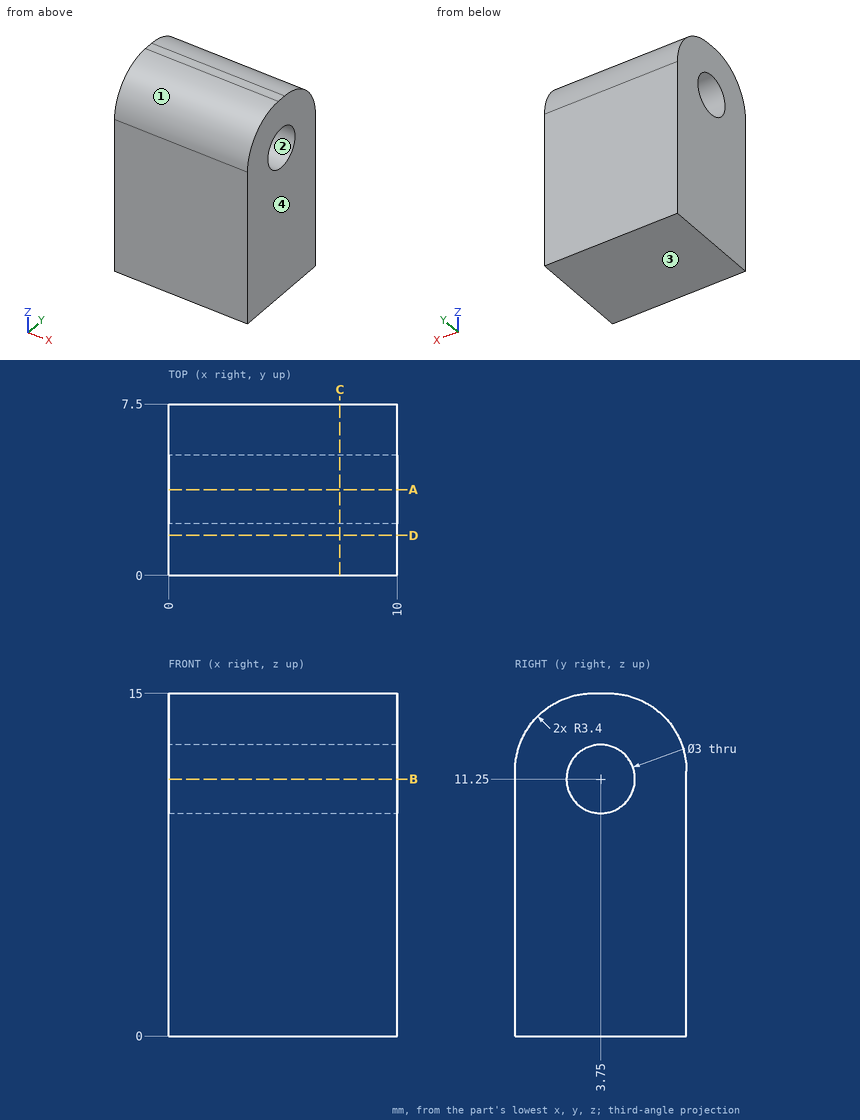
Here's the drawing with two shaded views (mm, measured from the low corner). I have some questions. Coordinates: 2 decimals unless noted, no trailing zeros. Order: outer loops, then holes, each group sorted by start corner. A loop starts at its lowest first (then second) coordinate and runs counter-clockwise, first axis right, second up.
Q1. Suppose I cut it at D-D on y = 1.75. Please give me the cut outline in (x, z).
Q2. Suppose I cut it at B-B on z = 11.25. Please give me the cut outline in (x, y), and give its area (3 significant figures).
Q3. Suppose I cut it at A-A on y = 3.75. Please give me the cut outline in (x, z).
Q4. Will this pin go through, and if not, where does the flat tip stop? pin 1 (1 mm diameter, centred on x = 4.5, y = 2.5, fed in from +Z).
Q5. Please list where these lines run through material, in increasing order: L1, parallel to Y at x = 7.75, z = 11.25; L2, parallel to Z at x = 7, y = 3.5; L3, parallel to Y at x = 7.5, z = 10.25.
Q6. Suppose I cut it at C-C on x = 7.5. Please give me the cut outline in (y, z), and give its area (3 significant figures).
Q7. Thinking about a two-plate mould opening in Z: for the marked faces 1, 2, 3 and 4, which applies, released by +Z, released by -Z, zero draft, split by the parting line, or undercut?
Answer:
1. outline: (0, 0) - (10, 0) - (10, 14.57) - (0, 14.57) - close
2. outline: (0, 0) - (10, 0) - (10, 2.25) - (0, 2.25) - close; (0, 5.25) - (10, 5.25) - (10, 7.5) - (0, 7.5) - close
2. area: 45.0 mm2
3. outline: (0, 0) - (10, 0) - (10, 9.75) - (0, 9.75) - close; (0, 12.75) - (10, 12.75) - (10, 15) - (0, 15) - close
4. pin 1: stops at z = 14.98
5. L1: y = 0 to 2.25, 5.25 to 7.5
5. L2: z = 0 to 9.77, 12.73 to 15
5. L3: y = 0 to 2.63, 4.87 to 7.5
6. outline: (0, 0) - (7.5, 0) - (7.5, 11.6) arc R3.4 ccw to (4.1, 15) - (3.4, 15) arc R3.4 ccw to (0, 11.6) - close; hole circle Ø3 at (3.75, 11.25)
6. area: 100 mm2
7. face 1: released by +Z
7. face 2: undercut
7. face 3: released by -Z
7. face 4: zero draft
